Can you work these out from the model? Positions are in its coordinate system, mm. A direction names the side the tool comes from. Round coordinates to 2 decimals unless told otherwise and drop trailing zeros. Loops run counter-clockwise (first coordinate to the right, second up) from the corner with the lowest first, then second, coordinate; pieces in that order, holes last. Notation, with made-up numbers: M 44.25,75 L 94.25,75 A15 ccw 94.25,99 Z; hole C 4,35 d6. An arc over 180 degrees is marked long. Return JSON: item names as keys, results as strings.
Autodesk Inventor part; units mm, degrees
ref_plane "YZ Plane" through (0, 0, 0) normal (1, 0, 0) x (0, 1, 0)
ref_plane "XZ Plane" through (0, 0, 0) normal (0, 1, 0) x (-1, 0, 0)
ref_plane "XY Plane" through (0, 0, 0) normal (0, 0, 1) x (1, 0, 0)
sketch "Sketch1" plane through (0, 0, 0) normal (1, 0, 0) x (0, 1, 0)
  line L0 (0, 0) -> (0, -38.1)
  line L1 (0, 0) -> (36.5125, 0)
  line L2 (36.5125, -51.0466) -> (36.5125, -57.15)
  line L3 (36.5125, -57.15) -> (35.1989, -57.15)
  line L4 (34.925, -50.8) -> (0, -38.1)
  line L5 (36.5125, -55.5625) -> (36.5125, -57.15)
  line L6 (36.5125, -55.5625) -> (36.1823, -55.5625)
  line L7 (36.1823, -55.5625) -> (36.1823, -51.2572)
  line L8 (36.1823, -55.5625) -> (40.5858, -55.5625) construction
  line L9 (34.925, -50.8) -> (36.1823, -51.2572)
  arc A0 (36.516, -55.6063) -> (36.5125, -55.5625) centre (35.0619, -55.6994) ccw
  line L10 (35.1989, -57.15) -> (36.1823, -55.5625)
  line L11 (0, 0) -> (0.3302, 0)
  line L12 (0.3302, 0) -> (0.1665, -37.8298)
  line L13 (36.1837, -50.927) -> (0.1665, -37.8298)
  line L14 (36.1837, -50.927) -> (36.5125, -51.0466)
  dimension "d0" = 38.1
  dimension "d1" = 36.5125
  dimension "d2" = 57.15
  dimension "d5" = 0.3302
  dimension "d6" = 90
  dimension "d7" = 0.3302
revolve "Revolution1" add sketch "Sketch1" angle 360 about axis through (0, 0, 0) along (0, 1, 0) contours L1 L12 L13 L14 L2 L6 L7 L9 L4 L0
properties part number "bowl-2" material "Stainless Steel"
Q1. I'm going to push flat-ended pins straight in: pin 1 Ø3 at (x, y) = (-36, 14.5) entering from +Z; pin 2 Ø1 at (y, z) = (29.5, 10) entering from -X; pin 3 Ø5 at (x, y) = (25.5, 11.5) entering from +Z. Where does each tip first touch, or does it pass through?
Results:
{"pin 1": "stops at z = 26.48", "pin 2": "stops at x = -48", "pin 3": "stops at z = 35.81"}
Q2. Suppose I cut it at B-B, the plane y = 31. Please give me the cut outline in (x, z).
Results:
{"outline": "C 0,0 d98.75; hole C 0,0 d98.08"}
Q3. Thinking about a two-plate mould opening in X: for faces 3 (the flat face through (45.01, 36.512, -24.44)), 4 (the conical face through (-1.44, 0.32, 1.88)), 5 (the conical face through (-11.691, 2.263, -37.126)), which applies, pulls with the +X half, pulls with the -X half, needs draft (parallel to the pull), parting line crosses it, or undercut?
Results:
{"face 3": "needs draft", "face 4": "undercut", "face 5": "parting line crosses it"}
Q4. On a 3-axis mill with a long thin cutter (end or side, diameter ignored), from which of +Z, -Z, +X, -X, +Y, -Y can I reach the whole of each face in a straight line? I mean faces 1 (the cylindrical face through (55.09, 36.35, 7.23)), 2 (the flat face through (49, 36.182, -16)). Say none if no direction works.
Results:
{"face 1": "+Y, -Y", "face 2": "-Y"}
Q5. If I drill on line 1 along Y through (x, z) = (-6, 33); line 2 along Y through (x, z) = (4, 4.5); line 3 along X through (y, z) = (34, 1.5), over which ranges is the centre line in solid material (lowest first)?
Results:
{"line 1": "y = 0 to 0.19", "line 2": "y = 0 to 0.3", "line 3": "x = -50.44 to -50.11, 50.11 to 50.44"}
Q6. Suppose I cut it at A-A, the plane y = 16. Please give me the cut outline in (x, z).
Results:
{"outline": "C 0,0 d87.84; hole C 0,0 d87.17"}
